Design review of the part shown in the three views and the two pictorial views. Dimensions are in mm from the part's minimum x, y and z. A direction names the side the tool comes from. Coordinates: 2 decimals unless noted, no trailing zeros. Write each loop counter-clockwise with the first axis right and the second up, starting at its lowest first coordinate (ties: lowest second). Pieces come first, ordered by that corner, then holes. Notation, with made-up numbers: (84.5, -13) -> (108.5, -13) arc R19 ccw to (108.5, 17) -> close; hole circle Ø9 at (53.5, 44). An arc over 180 degrees is marked (long way). Write item = value, one per line. Start each with the question number.
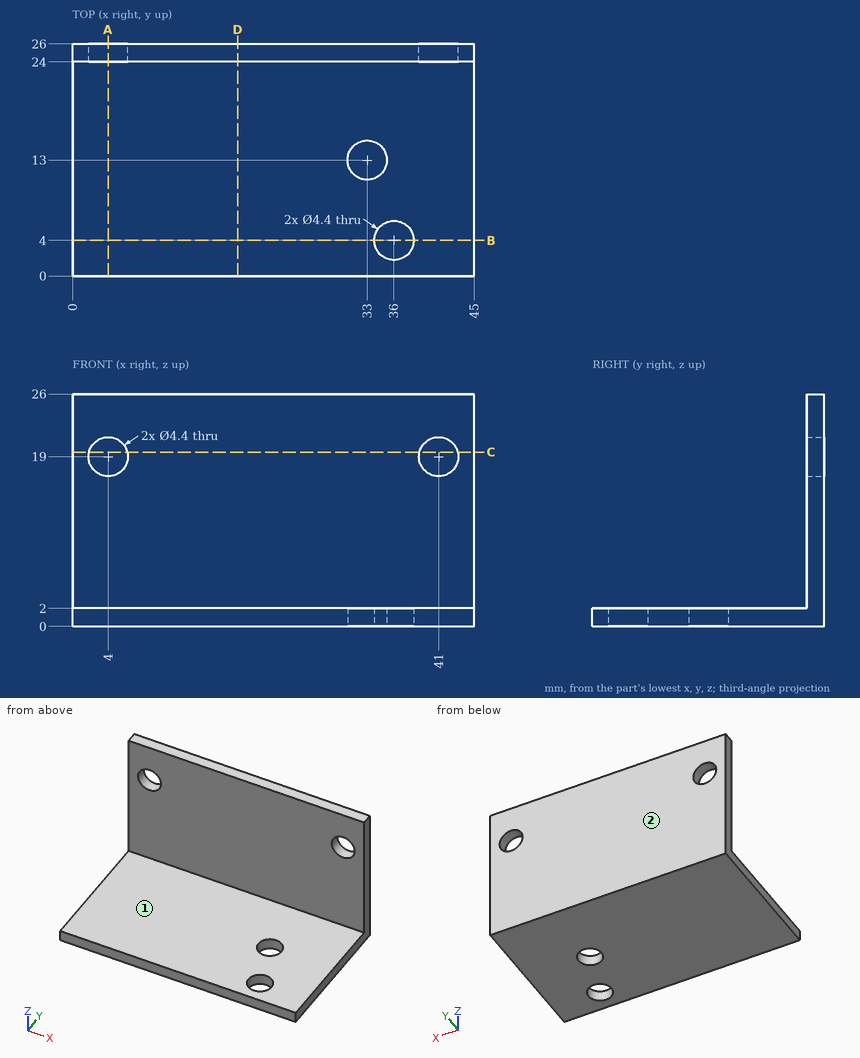
(1) For the marked faces 1 and 2, list the 3-axis set-ups (+Z, -Z, +X, -X, +Y, -Y) from which the entire face can be reached by the end or side of a thin tool; tool diameter is ignored.
(2) For line 1 (Y direction, x = 36, z = 0.85); line 2 (Y direction, x = 33, z = 1); line 3 (Z direction, x = 4, y = 25.05), list the stretches that pass through material, from the lowest coordinate up.
(3) Take a section at C-C, the plane z = 19.5. State the section outline as (x, y) points.
(4) Take a section at D-D, the plane x = 18.5. State the section outline as (y, z) points.
(5) For pin 1 Ø2.5 at (x, z) = (4, 19) entering from -Y; pin 2 Ø7 at (x, y) = (36, 4) entering from -Z; pin 3 Ø2 at (x, y) = (26, 16) entering from +Z; pin 4 Ø7 at (x, z) = (32.5, 19.5) entering from -Y, all flat-tipped, find the tip position at first contact; note any pin that passes through.
(6) Take a section at A-A, the plane x = 4. State the section outline as (y, z) points, then the cut area to 3 significant figures.
(7) Take a section at B-B, the plane y = 4. State the section outline as (x, z) points, then the cut area to 3 significant figures.
Report:
q1.face_1 = +Z, +X, -X, -Y
q1.face_2 = +Z, -Z, +X, -X, +Y
q2.line_1 = 0 to 1.8, 6.2 to 26
q2.line_2 = 0 to 10.8, 15.2 to 26
q2.line_3 = 0 to 16.8, 21.2 to 26
q3.outline = (0, 24) -> (1.86, 24) -> (1.86, 26) -> (0, 26) -> close; (6.14, 24) -> (38.86, 24) -> (38.86, 26) -> (6.14, 26) -> close; (43.14, 24) -> (45, 24) -> (45, 26) -> (43.14, 26) -> close
q4.outline = (0, 0) -> (26, 0) -> (26, 26) -> (24, 26) -> (24, 2) -> (0, 2) -> close
q5.pin_1 = through
q5.pin_2 = 0
q5.pin_3 = 2
q5.pin_4 = 24
q6.outline = (0, 0) -> (26, 0) -> (26, 16.8) -> (24, 16.8) -> (24, 2) -> (0, 2) -> close; (24, 21.2) -> (26, 21.2) -> (26, 26) -> (24, 26) -> close
q6.area = 91.2 mm2
q7.outline = (0, 0) -> (33.8, 0) -> (33.8, 2) -> (0, 2) -> close; (38.2, 0) -> (45, 0) -> (45, 2) -> (38.2, 2) -> close
q7.area = 81.2 mm2
